Autodesk Inventor part; units mm, degrees
ref_plane "Work Plane1" through (-108.8053, -23.2276, 20.9918) normal (0, 1, 0) x (-0.9999918, 0, -0.00406)
ref_plane "YZ Plane" through (0, 0, 0) normal (1, 0, 0) x (0, 1, 0)
ref_plane "XZ Plane" through (0, 0, 0) normal (0, 1, 0) x (-1, 0, 0)
ref_plane "Work Plane1" through (-108.8053, -23.2276, 20.9918) normal (0, 1, 0) x (-0.9999918, 0, -0.00406)
sketch "Sketch1" plane through (-108.8053, -23.2276, 20.9918) normal (0, 1, 0) x (-0.9999918, 0, -0.00406)
  line L0 (-46.787, -50.1863) -> (-47.193, 49.8137)
  line L1 (-47.193, 49.8137) -> (-40.843, 49.8137)
  line L2 (-46.787, -50.1863) -> (-40.437, -50.1863)
  line L3 (-46.787, -50.1863) -> (-40.437, -50.1863)
  line L4 (-40.843, 49.8137) -> (-40.437, -50.1863)
  line L5 (-47.193, 49.8137) -> (46.787, 50.1953) construction
  line L6 (-38.1849, 20.7247) -> (-38.1707, 17.2247)
  line L7 (-38.0296, -17.525) -> (-38.0154, -21.025)
  point P0 (-108.7192, -21.4334)
  dimension "d0" = 6.35
  dimension "d1" = 6.35
extrude "Extrusion1" add sketch "Sketch1" along normal blind 50.8 and the other way blind 6.35
sketch "Sketch2" plane through (-61.8149, -29.5776, 70.9967) normal (1, 0, 0) x (0, 0, -1)
  line L0 (100.0008, 0) -> (100.0008, 57.15) construction
  line L1 (0, 57.15) -> (100.0008, 57.15) construction
  line L2 (0, 0) -> (0, 57.15) construction
  line L3 (0, 57.15) -> (100.0008, 57.15) construction
  line L4 (50.0004, 57.15) -> (50.0004, 0) construction
  circle A0 centre (15.0004, 13.9978) radius 4
  circle A1 centre (85.0004, 13.9978) radius 4
  line L5 (40.4004, 9.271) -> (59.6004, 9.271)
  line L6 (59.6004, 9.271) -> (59.6004, 28.291)
  line L7 (59.6004, 28.291) -> (40.4004, 28.291)
  line L8 (40.4004, 28.291) -> (40.4004, 9.271)
  line L9 (21.3504, 9.271) -> (21.3504, 25.4) construction
  line L10 (21.3504, 20.3478) -> (13.3504, 20.3478) construction
  line L11 (21.3504, 9.271) -> (21.3504, 25.4)
  line L12 (78.6504, 9.271) -> (78.6504, 25.4)
  line L13 (11.1112, 0.635) -> (11.1112, 6.35)
  line L14 (22.2224, 6.35) -> (22.2224, 0.635)
  line L15 (33.3334, 0.635) -> (33.3334, 6.35)
  line L16 (44.4446, 6.35) -> (44.4446, 0.635)
  line L17 (55.5556, 0.635) -> (55.5556, 6.35)
  line L18 (66.6668, 6.35) -> (66.6668, 0.635)
  line L19 (88.8891, 6.35) -> (88.8891, 0.635)
  line L20 (77.7779, 0.635) -> (77.7779, 6.35)
  line L21 (0.0258, 0.635) -> (0.0258, 6.35) construction
  line L22 (0.0258, 57.15) -> (0.0258, 0.635) construction
  line L23 (88.8891, 0.635) -> (100.0266, 0.635)
  line L24 (100.0008, 6.35) -> (88.8891, 6.35)
  line L25 (77.7779, 0.635) -> (66.6668, 0.635)
  line L26 (66.6668, 6.35) -> (77.7779, 6.35)
  line L27 (55.5556, 0.635) -> (44.4446, 0.635)
  line L28 (44.4446, 6.35) -> (55.5556, 6.35)
  line L29 (33.3334, 0.635) -> (22.2224, 0.635)
  line L30 (22.2224, 6.35) -> (33.3334, 6.35)
  line L31 (11.1112, 0.635) -> (0.0258, 0.635)
  line L32 (11.1112, 6.35) -> (0.0258, 6.35)
  line L33 (0.0258, 0.635) -> (0.0258, 6.35)
  line L34 (100.0266, 0.635) -> (100.0008, 6.35)
  line L35 (59.6004, 9.271) -> (59.6004, 25.4)
  line L36 (40.4004, 9.271) -> (40.4004, 25.4)
  circle A2 centre (30.8754, 17.3) radius 1.75
  circle A3 centre (69.1254, 17.3) radius 1.75
  circle A4 centre (50.0004, 43.8624) radius 1.75
  point P0 (70.9967, 23.2276)
  point P1 (75.0381, 0)
  dimension "d9" = 8
  dimension "d10" = 8
  dimension "d13" = 35
  dimension "d14" = 8
  dimension "d26" = 5.715
  dimension "d27" = 5.715
  dimension "d28" = 5.715
  dimension "d29" = 5.715
  dimension "d30" = 5.715
extrude "Extrusion2" cut sketch "Sketch2" against normal blind 35
sketch "Sketch4" plane through (-108.8053, -29.5776, 20.9918) normal (0, -1, 0) x (0.9999918, 0, 0.00406)
  line L0 (46.787, -50.1863) -> (47.193, 49.8137)
  line L1 (47.193, 49.8137) -> (40.843, 49.8137)
  line L2 (40.843, 49.8137) -> (40.437, -50.1863)
  line L3 (40.437, -50.1863) -> (46.787, -50.1863)
  point P0 (108.7192, -21.4334)
extrude "Extrusion3" cut sketch "Sketch4" against normal up to surface (0.635 mm away)
equation "\"d27\" = d26"
equation "\"d28\" = d26"
equation "\"d29\" = d26"
equation "\"d30\" = d26"
equation "\"d11\" = d13"
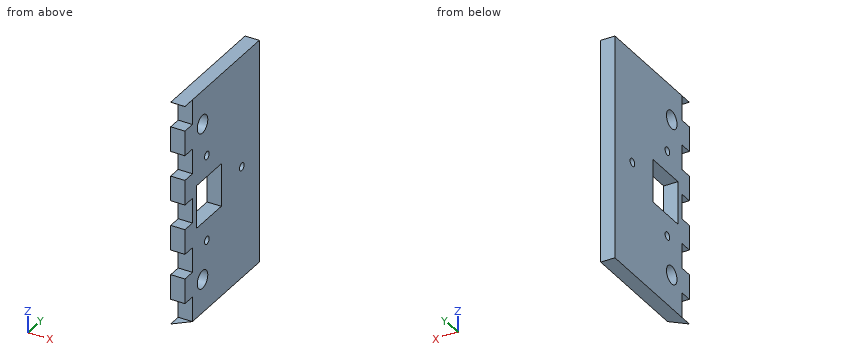
Verification items for the finished model (mm, model axes). Round coordinates to 2 decimals unless told otherwise and drop trailing zeros. Order: outer loops, then holes, each group sorted by start corner. A loop starts at its lowest first (then second) coordinate and runs counter-clockwise, first axis right, second up. Notation, with made-up numbers: (30, -12.5) - (47, -12.5) arc R30 ccw to (47, 24.5) - close; hole circle Ø4 at (-39, 19.25). An arc over 180 degrees is marked (long way). Use CSV: the item, a comma, the result in double quotes.
(1) Section check C-C on x = -64.5. State how many separate pieces and enclosed holes the cut face has, and give its area (3 significant figures).
Entries:
separate pieces,"1"
enclosed holes,"6"
area,"4,840 mm^2"
(2) Thickness scan on probe 1 along Y at (x, z) = (-66, 20.5); probe 2 along Y at (x, z) = (-65.5, 23); probe 3 along Z at (x, y) = (-65, -20). Record the ranges inside material, lowest first. Write a range as from..to.
Entries:
probe 1,"-23.23..-20.31, -1.29..12.61, 15.96..27.57"
probe 2,"-23.23..-20.31, -1.29..27.57"
probe 3,"-29.02..11.4, 30.6..70.98"
(3) Section check A-A on y = -3.5. Record the boundary of the cut face in (x, z), and give its area (3 significant figures).
Entries:
outline,"(-68.16, -29.03) - (-61.81, -29) - (-61.81, 11.4) - (-68.16, 11.4) - close; (-68.16, 30.6) - (-61.81, 30.6) - (-61.81, 71) - (-68.16, 70.97) - close"
area,"513 mm^2"
(4) Gauge pin test, flat ends, axial feed: pin 1 Ø9 at (y, z) = (-15.58, -14) entering from -X; pin 2 Ø3 at (x, z) = (-63.5, -22.5) entering from -Y; pin 3 Ø1.9 at (x, y) = (-65.5, -7.5) entering from -Z; pin 4 Ø3 at (x, y) = (-64.5, -27.5) entering from +Z. Record the tip position at first contact, or that the pin passes through.
Entries:
pin 1,"x = -68.16"
pin 2,"y = -23.23"
pin 3,"z = -29.02"
pin 4,"z = 70.99"
(5) Section check B-B on z = 24.5. Record the boundary of the cut face in (x, y), and give its area (3 significant figures).
Entries:
outline,"(-68.16, -23.23) - (-61.81, -23.23) - (-61.81, -20.31) - (-68.16, -20.31) - close; (-68.16, -1.29) - (-61.81, -1.29) - (-61.81, 27.57) - (-68.16, 27.57) - close"
area,"202 mm^2"
